from build123d import *

# Parameters (mm, degrees)
P_IDAT_VYSUNUT_M1_DEPTH       = 34.5
SKICA2_R                      = 1.5
ODEBRAT_VYSUNUT_M1_DEPTH      = 3
SKICA4_R                      = 1.75
ODEBRAT_VYSUNUT_M2_DEPTH      = 5
SKICA6_W                      = 3
SKICA6_H                      = 34.5
P_IDAT_VYSUNUT_M3_DEPTH       = 1.6
SKICA7_W                      = 3
SKICA7_H                      = 34.5
ODEBRAT_VYSUNUT_M3_DEPTH      = 1.6
ZAOBLIT1_R                    = 5
ZAOBLIT2_R                    = 5
ZAOBLIT3_R                    = 10
ZAOBLIT4_R                    = 5
ZAOBLIT5_R                    = 7
ZAOBLIT6_R                    = 14
ODEBRAT_VYSUNUT_M5_REACH      = 64.381
ODEBRAT_VYSUNUT_M5_END_RADIUS = 10
SKICA8_R                      = 3
SKICA9_R                      = 3
ODEBRAT_VYSUNUT_M6_DEPTH      = 3.5


with BuildPart() as part:
    # Skica1 → Přidat vysunutím1 (new body)
    with BuildSketch(Plane.XY):
        Polygon((0, 0), (38.660254038, 0), (47.320508076, 5), (31.570508076, 32.279800219), (34.168584287, 33.779800219), (59.168584287, -9.52146997), (56.570508076, -11.02146997), (49.820508076, 0.669872981), (40, -5), (0, -5), align=None)
    extrude(amount=P_IDAT_VYSUNUT_M1_DEPTH)

    # Skica2 → Odebrat vysunutím1 (cut)
    with BuildSketch(Plane(origin=(40.253520778, 23.240381057, 0), x_dir=(0, 0, -1), z_dir=(0.8660254037844362, 0.5000000000000046, 0))):
        with Locations(Location((-29.25, 5.769872981, 0), (0, 0, 90))):
            Circle(SKICA2_R)
        with Locations(Location((-29.25, -31.430127019, 0), (0, 0, 90))):
            Circle(SKICA2_R)
        with Locations(Location((-5.25, 5.769872981, 0), (0, 0, 90))):
            Circle(SKICA2_R)
        with Locations(Location((-5.25, -31.430127019, 0), (0, 0, 90))):
            Circle(SKICA2_R)
    extrude(amount=-ODEBRAT_VYSUNUT_M1_DEPTH, mode=Mode.SUBTRACT)

    # Skica4 → Odebrat vysunutím2 (cut)
    with BuildSketch(Plane(origin=(0, 0, 0), x_dir=(1, 0, 0), z_dir=(0, 1, 0))):
        with Locations(Location((6, -6, 0), (0, 0, 270))):
            Circle(SKICA4_R)
        with Locations(Location((6, -28.5, 0), (0, 0, 270))):
            Circle(SKICA4_R)
        with Locations(Location((24, -28.5, 0), (0, 0, 270))):
            Circle(SKICA4_R)
        with Locations(Location((24, -6, 0), (0, 0, 270))):
            Circle(SKICA4_R)
    extrude(amount=-ODEBRAT_VYSUNUT_M2_DEPTH, mode=Mode.SUBTRACT)

    # Skica6 → Přidat vysunutím3 (add)
    with BuildSketch(Plane(origin=(-6.084936491, 10.539419162, 0), x_dir=(0.8660254037844357, 0.5000000000000052, 0), z_dir=(-0.5000000000000052, 0.8660254037844357, 0))):
        with Locations((44.980762114, -17.25)):
            Rectangle(SKICA6_W, SKICA6_H)
    extrude(amount=P_IDAT_VYSUNUT_M3_DEPTH)

    # Skica7 → Odebrat vysunutím3 (cut)
    with BuildSketch(Plane(origin=(18.915063509, -32.761851027, 0), x_dir=(0.8660254037844368, 0.5000000000000032, 0), z_dir=(0.5000000000000032, -0.8660254037844368, 0))):
        with Locations((44.980762114, 17.25)):
            Rectangle(SKICA7_W, SKICA7_H)
    extrude(amount=-ODEBRAT_VYSUNUT_M3_DEPTH, mode=Mode.SUBTRACT)

    # Zaoblit1
    zaoblit1_edges = [part.edges().sort_by_distance(p)[0] for p in [
        (32.069546181, 34.415440865, 0),
        (32.069546181, 34.415440865, 34.5),
        (57.069546181, -8.885829324, 34.5),
        (57.069546181, -8.885829324, 0),
    ]]
    fillet(zaoblit1_edges, radius=ZAOBLIT1_R)

    # Zaoblit2
    zaoblit2_edges = [part.edges().sort_by_distance(p)[0] for p in [
        (0, -2.5, 0),
        (0, -2.5, 34.5),
    ]]
    fillet(zaoblit2_edges, radius=ZAOBLIT2_R)

    # Zaoblit3
    zaoblit3_edges = [part.edges().sort_by_distance(p)[0] for p in [
        (47.320508076, 5, 17.25),
    ]]
    fillet(zaoblit3_edges, radius=ZAOBLIT3_R - 0.0001)  # a hair under: the kernel refuses the full size

    # Zaoblit4
    zaoblit4_edges = [part.edges().sort_by_distance(p)[0] for p in [
        (49.820508076, 0.669872981, 17.25),
    ]]
    fillet(zaoblit4_edges, radius=ZAOBLIT4_R)

    # Zaoblit5
    zaoblit5_edges = [part.edges().sort_by_distance(p)[0] for p in [
        (38.660254038, 0, 17.25),
    ]]
    fillet(zaoblit5_edges, radius=ZAOBLIT5_R)

    # Zaoblit6
    zaoblit6_edges = [part.edges().sort_by_distance(p)[0] for p in [
        (40, -5, 17.25),
    ]]
    fillet(zaoblit6_edges, radius=ZAOBLIT6_R)

    # Odebrat vysunutím5: up to this cylinder (the profile starts outside it)
    odebrat_vysunut_m5_end = Plane(origin=(33.660254038, 8.660254038, 8.7), z_dir=(0, 0, 1)) * Cylinder(ODEBRAT_VYSUNUT_M5_END_RADIUS, 149.762, mode=Mode.PRIVATE)
    # Skica8 → Odebrat vysunutím5 (cut, up to the surface)
    with BuildSketch(Plane(origin=(40.253520778, 23.240381057, 0), x_dir=(0, 0, -1), z_dir=(0.8660254037844367, 0.5000000000000033, 0)), mode=Mode.PRIVATE) as odebrat_vysunut_m5_sk1:
        with Locations(Location((-8.7, -7.130127019, 0), (0, 0, 90))):
            Circle(SKICA8_R)
    odebrat_vysunut_m5_tool1 = extrude(odebrat_vysunut_m5_sk1.sketch, amount=-ODEBRAT_VYSUNUT_M5_REACH, mode=Mode.PRIVATE) - odebrat_vysunut_m5_end
    add(odebrat_vysunut_m5_tool1.solids().sort_by_distance((43.818584, 17.06551, 8.7))[0], mode=Mode.SUBTRACT)

    # Skica9 → Odebrat vysunutím6 (cut)
    with BuildSketch(Plane(origin=(40.253520778, 23.240381057, 0), x_dir=(0, 0, -1), z_dir=(0.8660254037844367, 0.5000000000000033, 0))):
        with Locations(Location((-8.7, -20.930127019, 0), (0, 0, 90))):
            Circle(SKICA9_R)
    extrude(amount=-ODEBRAT_VYSUNUT_M6_DEPTH, mode=Mode.SUBTRACT)


solid = part.part
Read the model definition and answer for the solid it produces. Units are mm, in the model's axes. A direction names the side the tool comes from. Coordinates: 2 decimals unless noted, no trailing zeros. Write each loop counter-clockwise with the first axis right and the second up, starting at its lowest first coordinate (ties: lowest second). Pieces come first, ordered by that corner, then holes. Notation, with made-up numbers: (71, 88.5) -> (83, 88.5) arc R23 ccw to (83, 106.5) -> close; hole circle Ø4 at (73.25, -22). An arc over 180 degrees is marked (long way). Return JSON: item names as keys, results as strings.
(1) The part is cut by section D-D on y = 9.5. Give the vertices of the cut face in (x, z), then the cut area to 3 significant figures.
Answers below:
{"outline": "(43.62, 0) -> (48.19, 0) -> (48.19, 34.5) -> (43.62, 34.5) -> close", "area": "157 mm^2"}
(2) For a pull along X with two mould halves and no side action, classify faces 1 (the cylindrical face through (56.336, -7.573, 33.074)), 2 (the flat face through (0, -3, 17)), 3 (the cylindrical face through (6.08, -2.46, 26.75)) as pulls with the +X half, pulls with the -X half, needs draft (parallel to the pull), parting line crosses it, or undercut.
Answers below:
{"face 1": "pulls with the +X half", "face 2": "pulls with the -X half", "face 3": "undercut"}
(3) Consider line 1 along X through (y, z) = (-2, 28); line 2 along X through (y, z) = (-3, 6); line 3 along X through (y, z) = (-1, 6). Determine where each line is inside the solid, lowest interval first. Write a range as from..to.
Answers below:
{"line 1": "0..4.32, 7.68..22.32, 25.68..45.2, 50.76..54.83", "line 2": "0..4.25, 7.75..22.25, 25.75..43.46, 51.87..55.07", "line 3": "0..4.25, 7.75..22.25, 25.75..54.25"}
(4) The part is cut by section C-C on z = 28.5. State how many separate pieces and enclosed holes the cut face has, then the cut area to 3 significant figures.
Answers below:
{"separate pieces": "5", "enclosed holes": "0", "area": "376 mm^2"}
(5) The part is cut by section A-A on x = 24. Give the vertices of the cut face in (y, z).
Answers below:
{"outline": "(-5, 0) -> (0, 0) -> (0, 4.25) -> (-5, 4.25) -> close; (-5, 7.75) -> (0, 7.75) -> (0, 26.75) -> (-5, 26.75) -> close; (-5, 30.25) -> (0, 30.25) -> (0, 34.5) -> (-5, 34.5) -> close"}
(6) Each of these flat-tipped pins is pushed along its axis until it touches: P1, Ø2, axis at y = 3, z = 19.5, coming from the -X side; P2, Ø10, axis at x = 45, z = 30.5, coming from the -Y side; P3, Ø4, axis at x = 24, z = 28.5, coming from the -Y side. Where does it stop, or does it pass through?
Answers below:
{"P1": "x = 41.06", "P2": "y = -4.49", "P3": "y = -5"}
(7) The part is cut by section B-B on x = 30. Give the vertices of the cut face in (y, z), then the cut area to 4 significant figures.
Answers below:
{"outline": "(-5, 0) -> (0, 0) -> (0, 34.5) -> (-5, 34.5) -> close", "area": "172.5 mm^2"}
(8) Which of the six approach directions +Z, -Z, +X, -X, +Y, -Y give full straight-line access (tool end or side, diameter ignored) to faces 4 (the flat face through (47.708, 3.328, 8.742)), 5 (the flat face through (44.385, -2.468, 17.008)), 6 (the flat face through (36, -1, 34.5))?
Answers below:
{"face 4": "none", "face 5": "+Z, -Z, -Y", "face 6": "+Z, +X, -X, +Y, -Y"}
